Work out the finished part from the listing and answer in its coordinate system (mm). Face numbers are marked on the shaded views. A direction names the side the tool comes from. Coordinates: 2 decimals unless noted, no trailing zeros. Order: outer loops, then holes, each group sorted by start corner. A loop starts at its lowest first (then second) coordinate and runs counter-clockwise, first axis right, second up. Notation, with made-up numbers: M 88.5,57 L 107.5,57 A30 ccw 107.5,87 Z; hole C -32.75,81 d3. An arc over 180 degrees is marked long. Use a Markdown table: item, result. Add a question column.
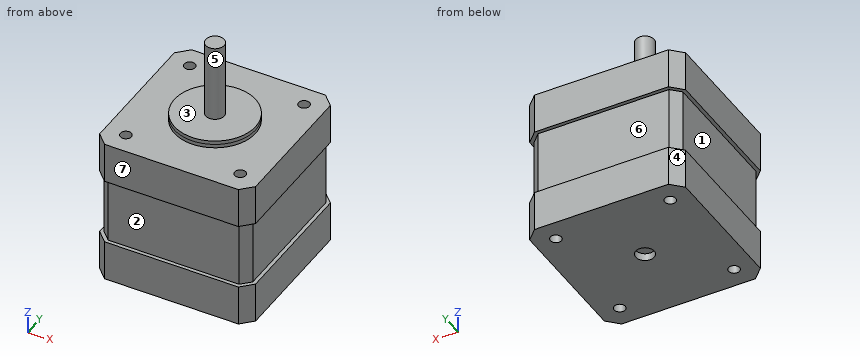
from build123d import *

# Parameters (mm, degrees)
EXTRUDE_1_DEPTH     = 10
SKETCH_2_R          = 11
EXTRUDE_2_DEPTH     = 2
SKETCH_3_R          = 2.5
EXTRUDE_3_DEPTH     = 22
EXTRUDE_4_DEPTH     = 18
EXTRUDE_5_DEPTH     = 10
SKETCH_4_R          = 1.5
CUT_EXTRUDE_1_DEPTH = 46.5
SKETCH_5_R          = 2.5
CUT_EXTRUDE_2_DEPTH = 1
SKETCH_9_R          = 1.5
EXTRUDE_6_DEPTH     = 1
SKETCH_10_R         = 1.5
SKETCH_10_R_2       = 2.5
EXTRUDE_7_DEPTH     = 1
SKETCH_11_R         = 11
SKETCH_11_R_2       = 2.5
EXTRUDE_8_DEPTH     = 1


with BuildPart() as part:
    # Эскиз1 → Бобышка-Вытянуть1 (new body)
    with BuildSketch(Plane.XY):
        Polygon((-32.767753805, -16.536194896), (-32.767753805, 19.763805104), (-29.767753805, 22.763805104), (6.532246195, 22.763805104), (9.532246195, 19.763805104), (9.532246195, -16.536194896), (6.532246195, -19.536194896), (-29.767753805, -19.536194896), align=None)
    extrude(amount=EXTRUDE_1_DEPTH)

    # Эскиз2 → Бобышка-Вытянуть2 (add)
    with BuildSketch(Plane.XY.offset(10)):
        with Locations(Location((-11.617753805, 1.613805104, 0), (0, 0, 180))):
            Circle(SKETCH_2_R)
    extrude(amount=EXTRUDE_2_DEPTH)

    # Эскиз3 → Бобышка-Вытянуть3 (add)
    with BuildSketch(Plane.XY.offset(12)):
        with Locations((-11.617753805, 1.613805104)):
            Circle(SKETCH_3_R)
    extrude(amount=EXTRUDE_3_DEPTH)

    # Эскиз6 → Бобышка-Вытянуть4 (add)
    with BuildSketch(Plane(origin=(0, 0, 0), x_dir=(-1, 0, 0), z_dir=(0, 0, -1))):
        Polygon((11.617753805, 21.763805104), (-6.118032632, 21.763805104), (-8.532246195, 19.349591542), (-8.532246195, -16.121981333), (-6.118032632, -18.536194896), (29.353540243, -18.536194896), (31.767753805, -16.121981333), (31.767753805, 19.349591542), (29.353540243, 21.763805104), align=None)
    extrude(amount=EXTRUDE_4_DEPTH)

    # Эскиз7 → Бобышка-Вытянуть5 (add)
    with BuildSketch(Plane.XY.offset(-18)):
        Polygon((-32.767753805, -16.536194896), (-32.767753805, 19.763805104), (-29.767753805, 22.763805104), (6.532246195, 22.763805104), (9.532246195, 19.763805104), (9.532246195, -16.536194896), (6.532246195, -19.536194896), (-29.767753805, -19.536194896), align=None)
    extrude(amount=-EXTRUDE_5_DEPTH)

    # Эскиз4 → Вырез-Вытянуть1 (cut)
    with BuildSketch(Plane.XY.offset(10)):
        with Locations((-27.117753805, 17.113805104)):
            Circle(SKETCH_4_R)
        with Locations((3.882246195, 17.113805104)):
            Circle(SKETCH_4_R)
        with Locations((3.882246195, -13.886194896)):
            Circle(SKETCH_4_R)
        with Locations((-27.117753805, -13.886194896)):
            Circle(SKETCH_4_R)
    extrude(amount=-CUT_EXTRUDE_1_DEPTH, mode=Mode.SUBTRACT)

    # Эскиз5 → Вырез-Вытянуть2 (cut)
    with BuildSketch(Plane(origin=(0, 0, -28), x_dir=(-1, 0, 0), z_dir=(0, 0, -1))):
        with Locations(Location((11.617753805, 1.613805104, 0), (0, 0, 180))):
            Circle(SKETCH_5_R)
    extrude(amount=-CUT_EXTRUDE_2_DEPTH, mode=Mode.SUBTRACT)

    # Эскиз9 → Бобышка-Вытянуть6 (add)
    with BuildSketch(Plane.XY.offset(10)):
        Polygon((-29.767753805, 22.763805104), (-32.767753805, 19.763805104), (-32.767753805, -16.536194896), (-29.767753805, -19.536194896), (6.532246195, -19.536194896), (9.532246195, -16.536194896), (9.532246195, 19.763805104), (6.532246195, 22.763805104), align=None)
        with Locations((3.882246195, 17.113805104)):
            Circle(SKETCH_9_R, mode=Mode.SUBTRACT)
        with Locations((3.882246195, -13.886194896)):
            Circle(SKETCH_9_R, mode=Mode.SUBTRACT)
        with Locations((-27.117753805, -13.886194896)):
            Circle(SKETCH_9_R, mode=Mode.SUBTRACT)
        with Locations((-27.117753805, 17.113805104)):
            Circle(SKETCH_9_R, mode=Mode.SUBTRACT)
    extrude(amount=EXTRUDE_6_DEPTH)

    # Эскиз10 → Бобышка-Вытянуть7 (add)
    with BuildSketch(Plane(origin=(0, 0, -28), x_dir=(-1, 0, 0), z_dir=(0, 0, -1))):
        Polygon((32.767753805, 19.763805104), (29.767753805, 22.763805104), (-6.532246195, 22.763805104), (-9.532246195, 19.763805104), (-9.532246195, -16.536194896), (-6.532246195, -19.536194896), (29.767753805, -19.536194896), (32.767753805, -16.536194896), align=None)
        with Locations(Location((-3.882246195, -13.886194896, 0), (0, 0, 180))):
            Circle(SKETCH_10_R, mode=Mode.SUBTRACT)
        with Locations(Location((27.117753805, -13.886194896, 0), (0, 0, 180))):
            Circle(SKETCH_10_R, mode=Mode.SUBTRACT)
        with Locations(Location((11.617753805, 1.613805104, 0), (0, 0, 180))):
            Circle(SKETCH_10_R_2, mode=Mode.SUBTRACT)
        with Locations(Location((-3.882246195, 17.113805104, 0), (0, 0, 180))):
            Circle(SKETCH_10_R, mode=Mode.SUBTRACT)
        with Locations(Location((27.117753805, 17.113805104, 0), (0, 0, 180))):
            Circle(SKETCH_10_R, mode=Mode.SUBTRACT)
    extrude(amount=EXTRUDE_7_DEPTH)

    # Эскиз11 → Бобышка-Вытянуть8 (add)
    with BuildSketch(Plane.XY.offset(12)):
        with Locations((-11.617753805, 1.613805104)):
            Circle(SKETCH_11_R)
        with Locations(Location((-11.617753805, 1.613805104, 0), (0, 0, 180))):
            Circle(SKETCH_11_R_2, mode=Mode.SUBTRACT)
    extrude(amount=EXTRUDE_8_DEPTH)


solid = part.part
(1) A cutting plane is placed at B-B on z = 8.5. Write down the section's boundary in (x, y).
(2) The mould has two halves that part along Z. Classify the marked faces 1, 2, 3 and 4: pulls with the +Z half, pulls with the -Z half, needs draft (parallel to the pull), parting line crosses it, or undercut.
(3) Which of the six approach directions +Z, -Z, +X, -X, +Y, -Y give full straight-line access (tool end or side, diameter ignored) to the marked faces 5, 6 and 7?
(4) A cutting plane is placed at D-D on z = -8. Write down the section's boundary in (x, y).
(5) Given P1, Ø4, axis at x = -25, y = -11.5, coming from the +Z side; P2, Ø8, axis at x = -11.62, y = 1.61, coming from the -Z side; P3, Ø5.5, axis at x = -4, z = -11, coming from the -Y side; P4, Ø1.5, axis at y = 7, z = 13, coming from the -X side, each flat-ended and moving along its own axis, determine where each tip first touches the part or whether it passes through.
(6) Straight lines are drawn through the part: line 1 (Y direction, x = 4, z = -16.5); line 2 (X direction, y = -13.5, z = 7.5); line 3 (X direction, y = -15, z = -6). For each, find the intervals that lie inside material, in ascending order.
(7) A cutting plane is placed at A-A on x = -10.5. Write down the section's boundary in (y, z), plus the area to 3 significant figures.
(8) A cutting plane is placed at C-C on y = -4.5. Write down the section's boundary in (x, z).
From the geometry:
| question | item | result |
|---|---|---|
| 1 | outline | M -32.77,-16.54 L -29.77,-19.54 L 6.53,-19.54 L 9.53,-16.54 L 9.53,19.76 L 6.53,22.76 L -29.77,22.76 L -32.77,19.76 Z; hole C -27.12,-13.89 d3; hole C -27.12,17.11 d3; hole C 3.88,-13.89 d3; hole C 3.88,17.11 d3 |
| 2 | face 1 | undercut |
| 2 | face 2 | undercut |
| 2 | face 3 | pulls with the +Z half |
| 2 | face 4 | needs draft |
| 3 | face 5 | +Z |
| 3 | face 6 | +X, -X, +Y |
| 3 | face 7 | +Z, -Z, +X, -X, -Y |
| 4 | outline | M -31.77,-16.12 L -29.35,-18.54 L 6.12,-18.54 L 8.53,-16.12 L 8.53,19.35 L 6.12,21.76 L -29.35,21.76 L -31.77,19.35 Z; hole C -27.12,-13.89 d3; hole C -27.12,17.11 d3; hole C 3.88,-13.89 d3; hole C 3.88,17.11 d3 |
| 5 | P1 | stops at z = 11 |
| 5 | P2 | stops at z = -29 |
| 5 | P3 | stops at y = -18.54 |
| 5 | P4 | stops at x = -21.59 |
| 6 | line 1 | y = -18.54 to -15.38, -12.39 to 15.62, 18.61 to 21.76 |
| 6 | line 2 | x = -32.77 to -28.57, -25.67 to 2.43, 5.33 to 9.53 |
| 6 | line 3 | x = -31.77 to -28.12, -26.11 to 2.88, 4.89 to 8.53 |
| 7 | outline | M -19.54,-29 L -0.62,-29 L -0.62,-27 L 3.85,-27 L 3.85,-29 L 22.76,-29 L 22.76,-18 L 21.76,-18 L 21.76,0 L 22.76,0 L 22.76,11 L 12.56,11 L 12.56,13 L 3.85,13 L 3.85,34 L -0.62,34 L -0.62,13 L -9.33,13 L -9.33,11 L -19.54,11 L -19.54,0 L -18.54,0 L -18.54,-18 L -19.54,-18 Z |
| 7 | area | 1,780 mm2 |
| 8 | outline | M -32.77,-29 L 9.53,-29 L 9.53,-18 L 8.53,-18 L 8.53,0 L 9.53,0 L 9.53,11 L -2.47,11 L -2.47,13 L -20.76,13 L -20.76,11 L -32.77,11 L -32.77,0 L -31.77,0 L -31.77,-18 L -32.77,-18 Z |
